```python
from build123d import *

# Parameters (mm, degrees)
F1_DEPTH = 13.081
F2_R     = 2.032
F3_DEPTH = 10.16
F5_DEPTH = 13.082
F7_R     = 2.032
F8_DEPTH = 3.048


with BuildPart() as f1:
    # F0 (on Front) → F1 (new body)
    with BuildSketch(Plane.XZ):
        with BuildLine():
            ThreePointArc((6.604, 0), (0, 6.604), (-6.604, 0))
            Line((-6.604, 0), (6.604, 0))
        make_face()
        with BuildLine():
            Line((6.604, 0), (-6.604, 0))
            ThreePointArc((-6.604, 0), (0, -6.604), (6.604, 0))
        make_face()
    extrude(amount=F1_DEPTH)

    # F2 (on face) → F3 (cut)
    with BuildSketch(Plane.XZ.offset(13.081)):
        with Locations((0, -2.54)):
            Circle(F2_R)
    extrude(amount=-F3_DEPTH, mode=Mode.SUBTRACT)

    # F4 (on face) → F5 (cut, through all)
    with BuildSketch(Plane.XZ.offset(13.081)):
        with BuildLine():
            ThreePointArc((6.096, 2.54), (0, 6.604), (-6.096, 2.54))
            Line((-6.096, 2.54), (6.096, 2.54))
        make_face()
    extrude(amount=-F5_DEPTH, mode=Mode.SUBTRACT)

    # F7 (on offset) → F8 (cut)
    with BuildSketch(Plane.XY.offset(-6.604)):
        with Locations((0, -5.08)):
            Circle(F7_R)
    extrude(amount=F8_DEPTH, mode=Mode.SUBTRACT)


solid = f1.part
```
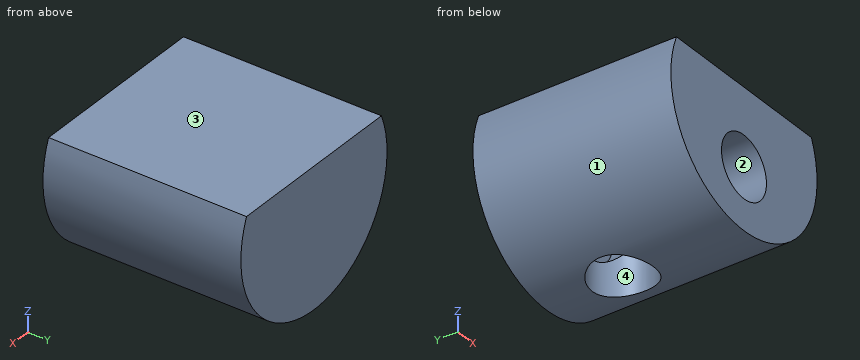
Work out the finished part from the listing and answer in its coordinate system (mm). Face numbers are marked on the shaded views. Coordinates: 2 decimals unless noted, no trailing zeros. Order: outer loops, then holes, each group sorted by start corner. A loop starts at its lowest first (then second) coordinate and runs counter-clockwise, first axis right, second up. Notation, with made-up numbers: (-5.5, -6.75) - (24.5, -6.75) arc R27 cw to (24.5, 21.25) - close; hole circle Ø5 at (36.25, 21). An arc over 180 degrees is marked (long way). Answer as a JSON object with one key per item and string values.
1. Find section C-C on z = -4.75. Determine the outline of the cut face in (x, y), plus the area to 3 significant figures.
Output values:
{"outline": "(-4.59, -13.08) - (4.59, -13.08) - (4.59, 0) - (-4.59, 0) - close; hole circle Ø4.06 at (0, -5.08)", "area": "107 mm²"}
2. Find section D-D on y = -9. Determine the outline of the cut face in (x, z).
Output values:
{"outline": "(-6.1, 2.54) arc R6.6 ccw (long way) to (6.1, 2.54) - close; hole circle Ø4.06 at (0, -2.54)"}
3. The mould has two halves that part along X. Classify the marked faces 1, 2, 3 and 4: +X half, -X half, draft (parallel to the pull), parting line (faces both ways), or undercut.
Output values:
{"face 1": "parting line", "face 2": "undercut", "face 3": "draft", "face 4": "undercut"}
4. Find section B-B on z = -2.54. Determine the outline of the cut face in (x, y).
Output values:
{"outline": "(-6.1, -13.08) - (-2.03, -13.08) - (-2.03, -2.92) - (2.03, -2.92) - (2.03, -13.08) - (6.1, -13.08) - (6.1, 0) - (-6.1, 0) - close"}
5. Consider line 1 (Y direction, x = 0, z = -5.6); line 2 (Z direction, x = 0, y = -9.25); line 3 (X direction, y = -7.25, z = -1). Determine where each line is inside the solid, lowest interval first.
Output values:
{"line 1": "y = -13.08 to -7.11, -3.05 to 0", "line 2": "z = -6.6 to -4.57, -0.51 to 2.54", "line 3": "x = -6.53 to -1.33, 1.33 to 6.53"}
6. Find section A-A on x = 0. Determine the outline of the cut face in (y, z).
Output values:
{"outline": "(-13.08, -6.6) - (-7.11, -6.6) - (-7.11, -4.57) - (-13.08, -4.57) - close; (-13.08, -0.51) - (-2.92, -0.51) - (-2.92, -4.57) - (-3.05, -4.57) - (-3.05, -6.6) - (0, -6.6) - (0, 2.54) - (-13.08, 2.54) - close"}
7. Each of these flat-tipped pins is pushed along its axis until it touches: P1, Ø2, axis at y = -11.5, z = -5, coming from the -X side; P2, Ø2, axis at x = -1.5, y = -7.5, coming from the -Z side; P3, Ø2, axis at y = -2, z = -2.5, coming from the +X side. Where does it stop, or does it pass through?
Output values:
{"P1": "stops at x = -5.25", "P2": "stops at z = -6.59", "P3": "stops at x = 6.43"}
